Part print with two shaded views. Sizes in mm from the minimum x, y, z corner. Coordinates: 2 decimals unless noted, no trailing zeros. Write each loop counter-clockwise with the first axis right and the second up, starting at its lowest first coordinate (ties: lowest second). Pieces come first, ordered by that corner, then holes. Notation, with made-up numbers: M 6,39.5 L 51,39.5 A33 ccw 51,69.5 Z; hole C 18,-6.5 d8. An arc over 180 degrees is marked long. Answer in a Markdown table with one row per item. Add a question column.
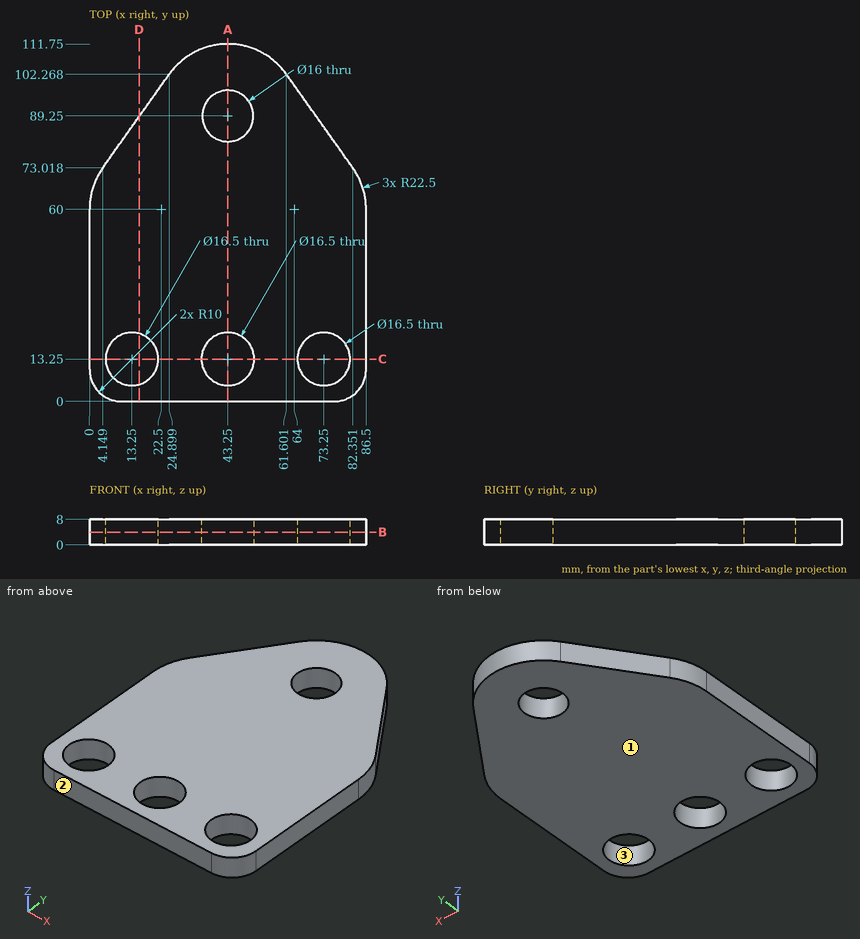
1) Drill centre lines: probe 1 along Y at (x, z) = (48, 4.25) (1 decimal); probe 2 along Y at (x, z) = (42.5, 4.75) (1 decimal); probe 3 along X at (y, z) = (16, 7.5). Where is each one in solid material? Low to high.
2) Two-plate mould, pull along Y, no slides. Class the marked faces 1, 2 and 3: released by +Y, released by -Y, zero draft, split by the parting line, or undercut.
3) Slice it at A-A (x = 43.25). Give the cut face in (y, z).
4) Slice it at B-B (z = 4). Give the cut face in (x, y), then the cut area to 3 significant figures.
5) Slice it at C-C (y = 13.25). Give the cut face in (x, z).
6) Slice it at D-D (x = 15.5). Give the cut face in (y, z), then the cut area to 3 significant figures.
7) Flat gauge pins, fed straight in: pin 1 Ø1 at (x, z) = (52, 6.5) entering from +Y; pin 2 Ø3 at (y, z) = (80, 3) entering from +X; pin 3 Ø2 at (x, z) = (32, 1.5) entering from +Y; pin 4 Ø9.5 at (x, y) = (43.25, 89.25) entering from -Z. Where does each tip first touch, or does it go through?
Ans:
| question | item | result |
|---|---|---|
| 1 | probe 1 | y = 0 to 6.5, 20 to 82.8, 95.7 to 111.2 |
| 1 | probe 2 | y = 0 to 5, 21.5 to 81.3, 97.2 to 111.7 |
| 1 | probe 3 | x = 0 to 5.47, 21.03 to 35.47, 51.03 to 65.47, 81.03 to 86.5 |
| 2 | face 1 | zero draft |
| 2 | face 2 | released by -Y |
| 2 | face 3 | undercut |
| 3 | outline | M 0,0 L 5,0 L 5,8 L 0,8 Z; M 21.5,0 L 81.25,0 L 81.25,8 L 21.5,8 Z; M 97.25,0 L 111.75,0 L 111.75,8 L 97.25,8 Z |
| 4 | outline | M 0,10 A10 ccw 10,0 L 76.5,0 A10 ccw 86.5,10 L 86.5,60 A22.5 ccw 82.35,73.02 L 61.6,102.27 A22.5 ccw 24.9,102.27 L 4.15,73.02 A22.5 ccw 0,60 Z; hole C 13.25,13.25 d16.5; hole C 43.25,13.25 d16.5; hole C 43.25,89.25 d16; hole C 73.25,13.25 d16.5 |
| 4 | area | 7,320 mm2 |
| 5 | outline | M 0,0 L 5,0 L 5,8 L 0,8 Z; M 21.5,0 L 35,0 L 35,8 L 21.5,8 Z; M 51.5,0 L 65,0 L 65,8 L 51.5,8 Z; M 81.5,0 L 86.5,0 L 86.5,8 L 81.5,8 Z |
| 6 | outline | M 0,0 L 5.31,0 L 5.31,8 L 0,8 Z; M 21.19,0 L 89.02,0 L 89.02,8 L 21.19,8 Z |
| 6 | area | 585 mm2 |
| 7 | pin 1 | stops at y = 110.18 |
| 7 | pin 2 | stops at x = 78.46 |
| 7 | pin 3 | stops at y = 109.28 |
| 7 | pin 4 | passes through |
